from build123d import *

# Parameters (mm, degrees)
SKETCH_1_W          = 120
SKETCH_1_H          = 120
EXTRUDE_1_DEPTH     = 2
SKETCH_2_R          = 2
SKETCH_2_R_2        = 1
EXTRUDE_2_DEPTH     = 15
SKETCH_3_W          = 53
SKETCH_3_H          = 18
SKETCH_3_W_2        = 45
SKETCH_3_W_3        = 14.5
SKETCH_3_W_4        = 7.5
SKETCH_3_H_2        = 13
SKETCH_3_H_3        = 89
CUT_EXTRUDE_3_DEPTH = 15
SKETCH_4_W          = 53
SKETCH_4_H          = 64
CUT_EXTRUDE_4_DEPTH = 15


with BuildPart() as part:
    # 스케치1 → 보스-돌출1 (new body)
    with BuildSketch(Plane(origin=(0, 0, 0), x_dir=(1, 0, 0), z_dir=(0, 1, 0))):
        Rectangle(SKETCH_1_W, SKETCH_1_H)
    extrude(amount=EXTRUDE_1_DEPTH)

    # 스케치2 → 보스-돌출2 (add)
    with BuildSketch(Plane(origin=(0, 2, 0), x_dir=(1, 0, 0), z_dir=(0, 1, 0))):
        with Locations(Location((55.5, 24.5, 0), (0, 0, 270))):
            Circle(SKETCH_2_R)
        with Locations(Location((55.5, -33.6, 0), (0, 0, 270))):
            Circle(SKETCH_2_R)
        with Locations(Location((48.5, -45.5, 0), (0, 0, 270))):
            Circle(SKETCH_2_R_2)
        with Locations(Location((22.5, -34, 0), (0, 0, 270))):
            Circle(SKETCH_2_R)
        with Locations(Location((22.5, 24.5, 0), (0, 0, 270))):
            Circle(SKETCH_2_R)
        with Locations(Location((48.5, 35.5, 0), (0, 0, 270))):
            Circle(SKETCH_2_R_2)
        with Locations(Location((-46, 34, 0), (0, 0, 270))):
            Circle(SKETCH_2_R_2)
        with Locations(Location((-44.5, -45.5, 0), (0, 0, 270))):
            Circle(SKETCH_2_R_2)
    extrude(amount=EXTRUDE_2_DEPTH)

    # 스케치3 → 컷-돌출3 (cut)
    with BuildSketch(Plane(origin=(0, 2, 0), x_dir=(1, 0, 0), z_dir=(0, 1, 0))):
        with Locations((-11.5, 51)):
            Rectangle(SKETCH_3_W, SKETCH_3_H)
        with Locations((37.5, 51)):
            Rectangle(SKETCH_3_W_2, SKETCH_3_H)
        with Locations((-45.25, 51)):
            Rectangle(SKETCH_3_W_3, SKETCH_3_H)
        with Locations((-56.25, 51)):
            Rectangle(SKETCH_3_W_4, SKETCH_3_H)
        with Locations((-56.25, 35.5)):
            Rectangle(SKETCH_3_W_4, SKETCH_3_H_2)
        with Locations((-56.25, -15.5)):
            Rectangle(SKETCH_3_W_4, SKETCH_3_H_3)
    extrude(amount=-CUT_EXTRUDE_3_DEPTH, mode=Mode.SUBTRACT)

    # 스케치4 → 컷-돌출4 (cut)
    with BuildSketch(Plane(origin=(0, 2, 0), x_dir=(1, 0, 0), z_dir=(0, 1, 0))):
        with Locations((-11.5, -28)):
            Rectangle(SKETCH_4_W, SKETCH_4_H)
    extrude(amount=-CUT_EXTRUDE_4_DEPTH, mode=Mode.SUBTRACT)


solid = part.part
Part model, mm, in its own coordinate system. A direction names the side the tool comes from. Coordinates: 2 decimals unless noted, no trailing zeros. Order: outer loops, then holes, each group sorted by start corner. A loop starts at its lowest first (then second) coordinate and runs counter-clockwise, first axis right, second up. Notation, with made-up numbers: M -10,-34.75 L 14,-34.75 A16 ccw 14,-13.75 Z; hole C -28.75,-10 d9. An arc over 180 degrees is marked long. One line per question, with ' | ' between items.
Q1. Slice it at D-D (z = -29). Give the cut face in (x, y).
A:
outline: M -52.5,0 L 60,0 L 60,2 L -52.5,2 Z
Q2. 3-axis set-ups, long thin cutter, end or side, ignore diameter. For faces 3 (the face through (57.483, 9.395, -24.76)), 4 (the face through (56, 17, -25)): which of +Z, -Z, +X, -X, +Y, -Y reach the whole face in a straight line?
A:
face 3: +Y | face 4: +Z, -Z, +X, -X, +Y
Q3. Slice it at B-B (x = 55.5). Give the cut face in (y, z), and give its area (3 significant figures).
A:
outline: M 0,-42 L 2,-42 L 2,-26.5 L 17,-26.5 L 17,-22.5 L 2,-22.5 L 2,31.6 L 17,31.6 L 17,35.6 L 2,35.6 L 2,60 L 0,60 Z | area: 324 mm^2
Q4. Slice it at C-C (z = 33.6). Give the cut face in (x, y).
A:
outline: M -52.5,0 L -38,0 L -38,2 L -52.5,2 Z; M 15,0 L 60,0 L 60,2 L 57.5,2 L 57.5,17 L 53.5,17 L 53.5,2 L 24.46,2 L 24.46,17 L 20.54,17 L 20.54,2 L 15,2 Z
Q5. Slice it at A-A (y = 11.5). Give the cut face in (x, z), and give its area (3 significant figures).
A:
outline: C -46,-34 d2; C -44.5,45.5 d2; C 22.5,-24.5 d4; C 22.5,34 d4; C 48.5,-35.5 d2; C 48.5,45.5 d2; C 55.5,-24.5 d4; C 55.5,33.6 d4 | area: 62.8 mm^2
Q6. Two-plate mould, pull along Z, no slides. Class faces 1 (the face through (21.3, 9.4, -26.1)), 2 (the face through (23, 17, 34)): +Z half, -Z half, draft (parallel to the pull), parting line (faces both ways), or undercut.
A:
face 1: undercut | face 2: draft
Q7. Pin check, flat tips, straight feed: P1, Ø0.6, axis at x = -3, y = 1.5, coming from the +Z side; P2, Ø3, axis at x = 25, z = 13.5, coming from the -Y side; P3, Ø8, axis at y = 8, z = 49, coming from the -X side; P4, Ø6, axis at y = 5.5, z = -6, coming from the +X side. Stop position of each tip, or through.
A:
P1: stops at z = -4 | P2: stops at y = 0 | P3: stops at x = -45.5 | P4: passes through
Q8. Drill centre lines: line 1 (Y direction, x = 41, z = 49); line 2 (X direction, y = 7.5, z = -35.5); line 3 (Z direction, x = 23.5, y = 16.75). Where is each one in solid material? Low to high.
A:
line 1: y = 0 to 2 | line 2: x = 47.5 to 49.5 | line 3: z = -26.23 to -22.77, 32.27 to 35.73
